Verification items for the finished model (mm, model axes). Face numbers are marked on the shaded views. A direction names the side the tool comes from. Round coordinates to 2 decimals unless told otherwise and drop trailing zeros. Write each loop counter-clockwise with the first axis right and the second up, starting at its lowest first coordinate (ties: lowest second). Pieces come first, ordered by that corner, then holes. Notation, with made-up numbers: M 42,58.5 L 52,58.5 A20 cw 52,83.5 Z; hole C 65.5,-22 d7. An arc over 180 degrees is marked long. One line per item, written item: value. Start each with the question number.
Item 1: Gauge pin test, flat ends, axial feed: pin 1 (10 mm diameter, centred on x = 9, y = -7, fed in from -Z); pin 2 (4 mm diameter, centred on x = 2.5, z = 4, fed in from -Y); pin 3 (3 mm diameter, centred on x = 9, z = 4, fed in from +Y). Record the tip position at first contact, or that the pin passes through.
Item 2: Draft check along Z on the marked faces 3, 4 and 5. Enter one of: +Z half, -Z half, draft (parallel to the pull), parting line (faces both ways), or undercut.
Item 3: Section check D-D, the plane x = 11.25. Record the cut outline in (y, z), then the cut area to 3 significant figures.
Item 4: Thickness scan on probe 1 along Z at (x, y) = (15, 4.25); probe 2 along Z at (x, y) = (10.25, 3.5); probe 3 along Y at (x, z) = (2.7, 0). Record the ranges inside material, lowest first. Write a range as from..to.
Item 5: Section check C-C, the plane x = 9.25. Record the cut outline in (y, z), then the cut area to 3 significant figures.
Item 6: Section check B-B, the plane x = 15.75. Record the cut outline in (y, z) (1 decimal), then the cut area to 3 significant figures.
Item 7: Tool access check on the marked faces 1 and 2. Record the directions out of +Z, -Z, +X, -X, +Y, -Y that give a thin tool (end or side, any length) a straight path to the whole face; none if there is none.
Autodesk Inventor part; units mm, degrees
ref_plane "YZ Plane" through (0, 0, 0) normal (1, 0, 0) x (0, 1, 0)
ref_plane "XZ Plane" through (0, 0, 0) normal (0, 1, 0) x (-1, 0, 0)
ref_plane "XY Plane" through (0, 0, 0) normal (0, 0, 1) x (1, 0, 0)
sketch "Sketch1" plane through (0, 0, 0) normal (0, 1, 0) x (-1, 0, 0)
  line L0 (0, 0) -> (-17.5, 0)
  line L1 (-17.5, 0) -> (-17.5, 5.7225) construction
  line L2 (-17.5, 8.5) -> (-12.5, 8.5)
  line L3 (-12.5, 8.5) -> (-12.5, 8.5)
  line L4 (-17.5, 8.5) -> (-17.5, 5.7225)
  line L5 (-12.5, 8.5) -> (-12.5, 8.5232)
  line L6 (-12.5, 8.5232) -> (0, 8.1326)
  line L7 (0, 8.1326) -> (0, 6.2)
  line L8 (-5.8333, 5.3579) -> (-17.5, 5.7225)
  line L9 (0, 6.2) -> (0, 0) construction
  line L10 (0, 6.2) -> (-5.8333, 6.2)
  line L11 (-5.8333, 6.2) -> (-5.8333, 5.3579)
  line L12 (-6.35, 8.331) -> (-6.35, 0) construction
  dimension "d0" = 11.445
  dimension "d1" = 17
  dimension "d4" = 17.5
  dimension "d5" = 5
  dimension "d7" = 1.79
  dimension "d9" = 12.4
  dimension "d10" = 5.8333
  dimension "d38" = 6.35
  dimension "d39" = 16.662
revolve "Revolve1" add sketch "Sketch1" angle 360 about axis through (0, 0, 0) along (1, 0, 0)
sketch "Sketch2" plane through (17.5, 0, 0) normal (1, 0, 0) x (0, 0, -1)
  circle A0 centre (0, 0) radius 8.5
  line L0 (-8.5, 4.9075) -> (0, 9.815)
  line L1 (0, 9.815) -> (8.5, 4.9075)
  line L2 (8.5, 4.9075) -> (8.5, -4.9075)
  line L3 (8.5, -4.9075) -> (0, -9.815)
  line L4 (0, -9.815) -> (-8.5, -4.9075)
  line L5 (-8.5, -4.9075) -> (-8.5, 4.9075)
  point P0 (-8.5, 0)
extrude "Extrude1" add sketch "Sketch2" against normal blind 5 contours L2 L3 A0 | A0 L1 L2 | A0 L0 L1 | L3 L4 A0 | A0 L5 L0 | L4 L5 A0
thread "Gwint1"
thread "Gwint2"
equation "\"d0\" = MD"
equation "\"d1\" = S"
equation "\"d4\" = L"
equation "\"d5\" = m1"
equation "\"d9\" = D3"
equation "\"d10\" = 0.333333 * L"
equation "\"d38\" = a"
equation "\"d39\" = MjD"
equation "\"d2\" = m1"
equation "\"MD\" = 11.445"
equation "\"m1\" = 5"
equation "\"S\" = 17"
equation "\"L\" = 17.5"
equation "\"D3\" = 12.4"
equation "\"a\" = 6.35"
equation "\"MjD\" = 16.662"
equation "\"a1\" = 3.7"
equation "\"Size_Designation\" = 1.2345"
properties part number "ISO 4145 Tuleja redukcyjna N4 3/8 x 1/4" material "Aluminium AW-7020"
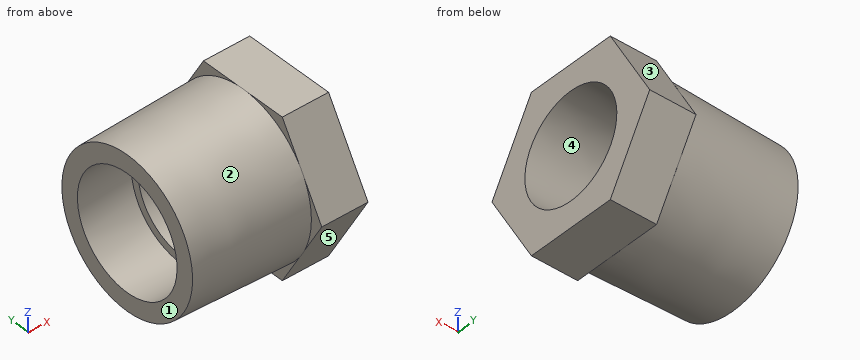
Response values:
1. pin 1: stops at z = -8.5
1. pin 2: stops at y = -7.97
1. pin 3: stops at y = 8.04
2. face 3: +Z half
2. face 4: undercut
2. face 5: -Z half
3. outline: C 0,0 d16.97; hole C 0,0 d11.05
3. area: 130 mm2
4. probe 1: z = -8.5..-3.71, 3.71..8.5
4. probe 2: z = -7.69..-4.24, 4.24..7.69
4. probe 3: y = -8.22..-6.2, 6.2..8.22
5. outline: C 0,0 d16.84; hole C 0,0 d10.93
5. area: 129 mm2
6. outline: M -9.8,0 L -4.9,-8.5 L 4.9,-8.5 L 9.8,0 L 4.9,8.5 L -4.9,8.5 Z; hole C 0,0 d11.3
6. area: 149 mm2
7. face 1: +Z, -Z, -X, +Y, -Y
7. face 2: -X
